The model under review builds one solid part; all positions refer to its coordinate system, in mm. A direction names the side the tool comes from. Coordinates: 2 decimals unless noted, no trailing zeros. Write each loop counter-clockwise with the first axis right and the second up, starting at its lowest first coordinate (ties: lowest second). Pieces come first, ordered by that corner, then holes.
1) Mouldability with a two-part tool opening along Z and no side actions: class faces 1 (the flat face through (45.35, 8, 0)), 2 (the flat face through (40.4, 4, 16.1)), 3 (the flat face through (-1, 8, 20.35)), 4 (the flat face through (43.35, 9, 0)) as released by +Z, released by -Z, zero draft, split by the parting line, or undercut.
2) Add section D-D, the plane y = 15. State the section outline as (x, z) points.
3) Machinability: for faces 5 (the cylindrical face through (38.063, 1.972, -14.745)), 6 (the flat face through (-44, 9, 6.185)), 7 (the flat face through (-1, 9, 18.35)), which of the approach directions +Z, -Z, +X, -X, +Y, -Y give a long, thin tool a straight path to every point of the face, cutting with its end or side? Answer none if there is none.
4) For P1, Ø4, axis at x = -13.5, z = -3, coming from the -Y side; P2, Ø3.5, axis at x = -39.55, z = 14.55, coming from the +Y side; P3, Ø4.5, axis at y = 11, z = -2, coming from the -X side; P4, Ø5, axis at x = 2.5, z = -4, coming from the +Y side, all flat-tipped, find the tip position at first contact; note any pin that passes through.
5) Add section C-C, the plane x = -39.55. State the section outline as (y, z) points, then the cut area to 3 significant figures.
6) Add section B-B, the plane z = 14.55. State the section outline as (x, y) points, then the cut area to 3 significant figures.
7) For line 1 (X direction, y = 2.7, z = 14.55); line 2 (Z direction, x = 39.55, y = 0.7); line 3 (X direction, y = 1.15, z = -14.55), list the stretches that pass through material, from the lowest coordinate up.
8) Add section A-A, the plane y = 3. State the section outline as (x, z) points.
from build123d import *

# Parameters (mm, degrees)
SKETCH1_W               = 90.7
SKETCH1_H               = 40.7
SKETCH1_R               = 1.5
BOSS_EXTRUDE3_DEPTH     = 2
SKETCH2_W               = 90.7
SKETCH2_H               = 40.7
SKETCH2_W_2             = 86.7
SKETCH2_H_2             = 36.7
BOSS_EXTRUDE4_DEPTH     = 15
CUT_EXTRUDE1_REACH      = 96.497
CUTOUT_W                = 12.369316876
CUTOUT_H                = 15
SKETCH3_R               = 1.5
BOSS_EXTRUDE5_DEPTH     = 2
MIRROR2_COPY_1_SKETCH_R = 1.5
MIRROR2_COPY_1_DEPTH    = 2


with BuildPart() as part:
    # Sketch1 → Boss-Extrude3 (new body)
    with BuildSketch(Plane(origin=(0, 0, 0), x_dir=(1, 0, 0), z_dir=(0, 1, 0))):
        Rectangle(SKETCH1_W, SKETCH1_H)
        with Locations(Location((-39.55, 14.55, 0), (0, 0, 270))):
            Circle(SKETCH1_R, mode=Mode.SUBTRACT)
        with Locations(Location((39.55, 14.55, 0), (0, 0, 270))):
            Circle(SKETCH1_R, mode=Mode.SUBTRACT)
        with Locations(Location((-39.55, -14.55, 0), (0, 0, 270))):
            Circle(SKETCH1_R, mode=Mode.SUBTRACT)
        with Locations(Location((39.55, -14.55, 0), (0, 0, 270))):
            Circle(SKETCH1_R, mode=Mode.SUBTRACT)
    extrude(amount=BOSS_EXTRUDE3_DEPTH)

    # Sketch2 → Boss-Extrude4 (add)
    with BuildSketch(Plane(origin=(0, 2, 0), x_dir=(1, 0, 0), z_dir=(0, 1, 0))):
        Rectangle(SKETCH2_W, SKETCH2_H)
        Rectangle(SKETCH2_W_2, SKETCH2_H_2, mode=Mode.SUBTRACT)
    extrude(amount=BOSS_EXTRUDE4_DEPTH)

    # Cutout → Cut-Extrude1 (cut, up to next)
    with BuildSketch(Plane.ZY.offset(45.35), mode=Mode.PRIVATE) as cut_extrude1_sk1:
        with Locations((0, 9.5)):
            Rectangle(CUTOUT_W, CUTOUT_H)
    cut_extrude1_tool1 = extrude(cut_extrude1_sk1.sketch, amount=-CUT_EXTRUDE1_REACH, mode=Mode.PRIVATE) & part.part
    add(cut_extrude1_tool1.solids().sort_by_distance((-45.35, 9.5, 0))[0], mode=Mode.SUBTRACT)

    # Sketch3 → Boss-Extrude5 (add)
    with BuildSketch(Plane(origin=(0, 2, 0), x_dir=(1, 0, 0), z_dir=(0, 1, 0))):
        with BuildLine():
            Line((-43.35, 12.35), (-38.35, 12.35))
            ThreePointArc((-38.35, 12.35), (-37.642893219, 12.642893219), (-37.35, 13.35))
            Line((-37.35, 13.35), (-37.35, 18.35))
            Line((-37.35, 18.35), (-43.35, 18.35))
            Line((-43.35, 18.35), (-43.35, 12.35))
        make_face()
        with Locations(Location((-39.55, 14.55, 0), (0, 0, 270))):
            Circle(SKETCH3_R, mode=Mode.SUBTRACT)
    boss_extrude5 = extrude(amount=BOSS_EXTRUDE5_DEPTH)

    # Mirror1: Boss-Extrude5 across plane
    add(boss_extrude5.mirror(Plane(origin=(0, 0, 0), x_dir=(0, 0, 1), z_dir=(1, 0, 0))))

    # Mirror2: Boss-Extrude5 across plane
    add(boss_extrude5.mirror(Plane.XY))

    # Mirror2 copy 1 sketch → Mirror2 copy 1 (add)
    with BuildSketch(Plane(origin=(0, 2, 0), x_dir=(-1, 0, 0), z_dir=(0, 1, 0))):
        with BuildLine():
            Line((-43.35, 12.35), (-38.35, 12.35))
            ThreePointArc((-38.35, 12.35), (-37.642893219, 12.642893219), (-37.35, 13.35))
            Line((-37.35, 13.35), (-37.35, 18.35))
            Line((-37.35, 18.35), (-43.35, 18.35))
            Line((-43.35, 18.35), (-43.35, 12.35))
        make_face()
        with Locations(Location((-39.55, 14.55, 0), (0, 0, 270))):
            Circle(MIRROR2_COPY_1_SKETCH_R, mode=Mode.SUBTRACT)
    extrude(amount=MIRROR2_COPY_1_DEPTH)


solid = part.part
Geometry results:
1. face 1: zero draft
1. face 2: undercut
1. face 3: released by +Z
1. face 4: undercut
2. outline: (-45.35, -20.35) - (45.35, -20.35) - (45.35, 20.35) - (-45.35, 20.35) - (-45.35, 6.18) - (-43.35, 6.18) - (-43.35, 18.35) - (43.35, 18.35) - (43.35, -18.35) - (-43.35, -18.35) - (-43.35, -6.18) - (-45.35, -6.18) - close
3. face 5: +Y, -Y
3. face 6: -X, +Y
3. face 7: +Y
4. P1: stops at y = 0
4. P2: stops at y = 4
4. P3: stops at x = 43.35
4. P4: stops at y = 2
5. outline: (0, -20.35) - (17, -20.35) - (17, -18.35) - (4, -18.35) - (4, -16.05) - (0, -16.05) - close; (0, -13.05) - (4, -13.05) - (4, -12.35) - (2, -12.35) - (2, 12.35) - (4, 12.35) - (4, 13.05) - (0, 13.05) - close; (0, 16.05) - (4, 16.05) - (4, 18.35) - (17, 18.35) - (17, 20.35) - (0, 20.35) - close
5. area: 141 mm2
6. outline: (-45.35, 0) - (-41.05, 0) - (-41.05, 4) - (-43.35, 4) - (-43.35, 17) - (-45.35, 17) - close; (-38.05, 0) - (38.05, 0) - (38.05, 4) - (37.35, 4) - (37.35, 2) - (-37.35, 2) - (-37.35, 4) - (-38.05, 4) - close; (41.05, 0) - (45.35, 0) - (45.35, 17) - (43.35, 17) - (43.35, 4) - (41.05, 4) - close
6. area: 241 mm2
7. line 1: x = -45.35 to -41.05, -38.05 to -37.35, 37.35 to 38.05, 41.05 to 45.35
7. line 2: z = -20.35 to -16.05, -13.05 to 13.05, 16.05 to 20.35
7. line 3: x = -45.35 to -41.05, -38.05 to 38.05, 41.05 to 45.35
8. outline: (-45.35, -20.35) - (45.35, -20.35) - (45.35, 20.35) - (-45.35, 20.35) - (-45.35, 6.18) - (-43.35, 6.18) - (-43.35, 12.35) - (-38.35, 12.35) arc R1 ccw to (-37.35, 13.35) - (-37.35, 18.35) - (37.35, 18.35) - (37.35, 13.35) arc R1 ccw to (38.35, 12.35) - (43.35, 12.35) - (43.35, -12.35) - (38.35, -12.35) arc R1 ccw to (37.35, -13.35) - (37.35, -18.35) - (-37.35, -18.35) - (-37.35, -13.35) arc R1 ccw to (-38.35, -12.35) - (-43.35, -12.35) - (-43.35, -6.18) - (-45.35, -6.18) - close; hole circle Ø3 at (-39.55, -14.55); hole circle Ø3 at (-39.55, 14.55); hole circle Ø3 at (39.55, -14.55); hole circle Ø3 at (39.55, 14.55)
